Work out the finished part from the listing and answer in its coordinate system (mm). A direction names the side the tool comes from. Coordinates: 2 decimals unless noted, no trailing zeros. Order: outer loops, then holes, each group sorted by start corner. A loop starts at its lowest first (then second) coordinate and runs counter-clockwise, first axis right, second up. Notation, with made-up numbers: (19.25, 31) -> (40.25, 31) arc R34 cw to (40.25, 62) -> close; hole circle Ø6 at (-14.5, 54). An arc over 180 degrees is marked (long way). Answer as CSV lines item,"result". Start each with the question number.
Item 1: For a pull along X with two mould halves and no side action, classify faces 1 (the face through (54.901, -14.498, 1.521)), 2 (the face through (-34, 134, 2)), 3 (the face through (-1, 22, 0)) as pulls with the +X half, pulls with the -X half, needs draft (parallel to the pull), parting line crosses it, or undercut.
Item 2: This flat-tipped pin is pushed along its axis until it touches: pin 1 Ø3 at (x, y) = (57.5, 8.5) entering from +Z. Where does it stop, or does it pass through?
Item 3: Which of the six approach directions +Z, -Z, +X, -X, +Y, -Y give full straight-line access (tool end or side, diameter ignored) to faces 4 (the face through (-54.901, 14.498, 1.521)), 5 (the face through (-87.482, 87.871, 1.521))?
Item 4: Section A-A (y = 7.5) is taken. Write down the section's boundary in (x, z).
Item 5: Straight lines are drawn through the part: L1, parallel to Y at x = 29, z = 1.9; L2, parallel to Y at x = -70, z = 0.25; L3, parallel to X at y = -6, z = 1.4. For each, find the intervals that lie inside material, in ascending order.
Item 6: Section B-B (z = 0.85) is taken. Count the separate pieces of the cut face and the enclosed holes in it, then the cut area to 3 significant figures.
Autodesk Inventor part; units mm, degrees
ref_plane "YZ Plane" through (0, 0, 0) normal (1, 0, 0) x (0, 1, 0)
ref_plane "XZ Plane" through (0, 0, 0) normal (0, 1, 0) x (-1, 0, 0)
ref_plane "XY Plane" through (0, 0, 0) normal (0, 0, 1) x (1, 0, 0)
sketch "Sketch1" plane through (0, 0, 0) normal (0, 0, 1) x (1, 0, 0)
  point P0 (0, 0)
sketch "Sketch2" plane through (0, 0, 0) normal (0, 0, 1) x (1, 0, 0)
  line L0 (94.9998, -95.0001) -> (-94.9998, -95.0001)
  line L1 (-94.9998, -95.0001) -> (-94.9998, 95.0001)
  line L2 (-94.9998, 95.0001) -> (94.9998, 95.0001)
  line L3 (94.9998, 95.0001) -> (94.9998, -95.0001)
  line L4 (94.9998, -95.0001) -> (-94.9998, 95.0001) construction
  line L5 (-94.9998, -95.0001) -> (94.9998, 95.0001) construction
  line L6 (-36.0001, 94.9999) -> (36.0001, 94.9999)
  line L7 (36.0001, 94.9999) -> (36.0001, 135.0001)
  line L8 (36.0001, 135.0001) -> (-36.0001, 135.0001)
  line L9 (-36.0001, 135.0001) -> (-36.0001, 94.9999)
  line L10 (-36.0001, 94.9999) -> (36.0001, 135.0001) construction
  line L11 (36.0001, 94.9999) -> (-36.0001, 135.0001) construction
  point P0 (0, 115)
  point P1 (-36.0001, 95.0001)
  point P2 (36.0001, 95.0001)
extrude "Extrusion1" add sketch "Sketch2" along normal blind 3
fillet "Fillet5" radius 25 4 edges at (-94.9998, 95.0001, 1.5) (94.9998, 95.0001, 1.5) (-94.9998, -95.0001, 1.5) (94.9998, -95.0001, 1.5)
fillet "Fillet6" radius 5 2 edges at (-36.0001, 135.0001, 1.5) (36.0001, 135.0001, 1.5)
sketch "Large Hammond mount holes" plane through (0, 0, 3) normal (0, 0, 1) x (1, 0, 0)
  circle A0 centre (16, 37) radius 2.0001
  circle A1 centre (-20, 123) radius 2.0001
  circle A2 centre (-20, 83) radius 2.0001
  circle A3 centre (16, 37) radius 2.0001
  circle A4 centre (-20, 123) radius 2.0001
  circle A5 centre (-20, 83) radius 2.0001
sketch "PX4FLOW mount holes" plane through (0, 0, 0) normal (0, 0, -1) x (-1, 0, 0)
  circle A0 centre (25.0336, 123.3517) radius 1.5872
  circle A1 centre (1.2211, 123.3517) radius 1.5872
  circle A2 centre (1.2211, 123.3517) radius 1.5872
  circle A3 centre (1.2211, 93.1892) radius 1.5872
  circle A4 centre (25.0336, 93.1892) radius 1.5872
sketch "Imperial standoffs" plane through (0, 0, 0) normal (0, 0, -1) x (-1, 0, 0)
  circle A0 centre (80, 80) radius 1.43
  circle A1 centre (-80, 80) radius 1.43
  circle A2 centre (-80, -80) radius 1.43
  circle A3 centre (80, -80) radius 1.43
extrude "Extrusion5" cut sketch "PX4FLOW mount holes" against normal blind 10
extrude "Extrusion7" cut sketch "Imperial standoffs" against normal blind 10
sketch "Dual pol balun cutout" plane through (0, 0, 3) normal (0, 0, 1) x (1, 0, 0)
  line L0 (26.2, -19.4999) -> (-26.2, -19.4999)
  line L1 (-26.2, -19.4999) -> (-26.2, 19.4999)
  line L2 (-26.2, 19.4999) -> (26.2, 19.4999)
  line L3 (26.2, 19.4999) -> (26.2, -19.4999)
  line L4 (26.2, -19.4999) -> (-26.2, 19.4999) construction
  line L5 (-26.2, -19.4999) -> (26.2, 19.4999) construction
  point P0 (0, 0)
extrude "Extrusion8" cut sketch "Dual pol balun cutout" against normal blind 10
sketch "SONAR_holes" plane through (0, 0, 3) normal (0, 0, 1) x (1, 0, 0)
  circle A0 centre (-8.501, 105) radius 1.6502
  circle A1 centre (8.519, 117.95) radius 1.6502
extrude "Extrusion9" cut sketch "SONAR_holes" against normal blind 10
sketch "SONAR cutouts" plane through (0, 0, 3) normal (0, 0, 1) x (1, 0, 0)
  line L0 (-55.0003, -9.9996) -> (-55.0003, 9.9996) construction
  line L1 (-50.5008, -9.9996) -> (-50.5008, 9.9996)
  line L2 (-59.4997, 9.9996) -> (-59.4997, -9.9996)
  arc A0 (-59.4997, -9.9996) -> (-50.5008, -9.9996) centre (-55.0003, -9.9996) ccw
  arc A1 (-50.5008, 9.9996) -> (-59.4997, 9.9996) centre (-55.0003, 9.9996) ccw
  line L3 (54.9997, -9.9996) -> (54.9997, 9.9996) construction
  line L4 (59.4992, -9.9996) -> (59.4992, 9.9996)
  line L5 (50.5003, 9.9996) -> (50.5003, -9.9996)
  arc A2 (50.5003, -9.9996) -> (59.4992, -9.9996) centre (54.9997, -9.9996) ccw
  arc A3 (59.4992, 9.9996) -> (50.5003, 9.9996) centre (54.9997, 9.9996) ccw
  point P0 (0, 0)
  point P1 (-55.0003, 0)
  point P2 (54.9997, 0)
extrude "Extrusion10" cut sketch "SONAR cutouts" against normal blind 10
sketch "Guard rails mount" plane through (0, 0, 0) normal (0, 0, -1) x (-1, 0, 0)
  circle A0 centre (-57.8735, 68.1265) radius 1.2499
  circle A1 centre (-68.1265, 57.8735) radius 1.2499
  circle A2 centre (57.8735, 68.1265) radius 1.2501
  circle A3 centre (68.1265, 57.8735) radius 1.2501
  circle A4 centre (-68.1265, -57.8735) radius 1.2501
  circle A5 centre (-57.8735, -68.1265) radius 1.2501
  circle A6 centre (57.8735, -68.1265) radius 1.2501
  circle A7 centre (68.1265, -57.8735) radius 1.2501
  circle A8 centre (-29.8735, 40.1265) radius 1.25
  circle A9 centre (-40.1265, 29.8735) radius 1.25
  circle A10 centre (40.1265, -29.8735) radius 1.25
  circle A11 centre (29.8735, -40.1265) radius 1.25
  circle A12 centre (29.8735, 40.1265) radius 1.25
  circle A13 centre (40.1265, 29.8735) radius 1.25
  circle A14 centre (-40.1265, -29.8735) radius 1.25
  circle A15 centre (-29.8735, -40.1265) radius 1.25
extrude "Extrusion12" cut sketch "Large Hammond mount holes" against normal blind 10
sketch "RPi mount holes" plane through (0, 0, 3) normal (0, 0, 1) x (1, 0, 0)
  circle A0 centre (29, -35.5) radius 1.2502
  circle A1 centre (29, -84.5) radius 1.2502
  circle A2 centre (-29, -35.5) radius 1.2502
  circle A3 centre (-29, -84.5) radius 1.2502
extrude "Extrusion14" cut sketch "RPi mount holes" against normal blind 10
sketch "balun_support_holes" plane through (0, 0, 3) normal (0, 0, 1) x (1, 0, 0)
  circle A0 centre (0, 0) radius 2.1823
  circle A1 centre (33.74, 25.4) radius 2.1823
  circle A2 centre (33.74, -25.4) radius 2.1823
  circle A3 centre (-33.74, 25.4) radius 2.1823
  circle A4 centre (-33.74, -25.4) radius 2.1823
extrude "Extrusion15" cut sketch "balun_support_holes" against normal blind 10 contours A1 | A2 | A3 | A4
sketch "Sketch20" plane through (0, 0, 0) normal (0, 0, -1) x (-1, 0, 0)
  circle A0 centre (-5.1265, 5.1265) radius 1.2502
  circle A1 centre (5.1265, -5.1265) radius 1.2502
  circle A2 centre (44.1265, -33.8735) radius 1.2502
  circle A3 centre (33.8735, -44.1265) radius 1.2502
  circle A4 centre (80.1265, -69.8735) radius 1.2502
  circle A5 centre (69.8735, -80.1265) radius 1.2502
  circle A6 centre (-33.8735, 44.1265) radius 1.2502
  circle A7 centre (-44.1265, 33.8735) radius 1.2502
  circle A8 centre (-69.8735, 80.1265) radius 1.2502
  circle A9 centre (-80.1265, 69.8735) radius 1.2502
  circle A10 centre (33.8735, 44.1265) radius 1.2502
  circle A11 centre (44.1265, 33.8735) radius 1.2502
  circle A12 centre (69.8735, 80.1265) radius 1.2502
  circle A13 centre (80.1265, 69.8735) radius 1.2502
  circle A14 centre (-44.1265, -33.8735) radius 1.2502
  circle A15 centre (-33.8735, -44.1265) radius 1.2502
  circle A16 centre (-80.1265, -69.8735) radius 1.2502
  circle A17 centre (-69.8735, -80.1265) radius 1.2502
extrude "Extrusion17" cut sketch "Sketch20" against normal blind 10 contours A2 | A3 | A4 | A5 | A6 | A7 | A8 | A9 | A10 | A11 | A12 | A13 | A14 | A15 | A16 | A17
properties part number "payload_bay_square_dual_pol_balun_v2" material "CFRP"
Checked values:
1,face 1,"undercut"
1,face 2,"pulls with the -X half"
1,face 3,"needs draft"
2,pin 1,"passes through"
3,face 4,"+Z, -Z"
3,face 5,"+Z, -Z, -X, +Y"
4,outline,"(-95, 0) -> (-59.5, 0) -> (-59.5, 3) -> (-95, 3) -> close; (-50.5, 0) -> (-26.2, 0) -> (-26.2, 3) -> (-50.5, 3) -> close; (26.2, 0) -> (50.5, 0) -> (50.5, 3) -> (26.2, 3) -> close; (59.5, 0) -> (95, 0) -> (95, 3) -> (59.5, 3) -> close"
5,L1,"y = -95 to -85.75, -83.25 to -36.75, -34.25 to 135"
5,L2,"y = -95 to -81.37, -78.88 to 78.88, 81.37 to 95"
5,L3,"x = -95 to -59.5, -50.5 to -26.2, 26.2 to 50.5, 59.5 to 95"
6,separate pieces,"1"
6,enclosed holes,"40"
6,area,"35,600 mm^2"
